Part model, mm, in its own coordinate system. Face numbers are marked on the shaded views. A direction names the side the tool comes from. Coordinates: 2 decimals unless noted, no trailing zeros. Loops run counter-clockwise (first coordinate to the right, second up) from the corner with the lowest first, then second, coordinate; pieces in that order, holes last. Notation, with made-up numbers: M 22,-28 L 52,-28 A20 ccw 52,1 Z; hole C 39.25,39 d5. An arc over 180 degrees is marked long. Use a Markdown table: item, result. Add a question column.
1) Pin check, flat tips, straight feed: pin 1 Ø1 at (y, z) = (-180, -95.5) entering from -X; pin 2 Ø12 at (y, z) = (-118.5, -103) entering from +X; pin 3 Ø14 at (x, y) = (-146, -101.5) entering from +Z. Stop position of each tip, or through.
2) Pull direction Z, two halves, no side cores. Call the marked faces 4, 5 and 6: released by +Z, released by -Z, zero draft, split by the parting line, or undercut.
3) Tool access for the marked faces 1, 2 and 3: list every direction of +Z, -Z, +X, -X, +Y, -Y with a clear straight run to the whole face (end or side of a thin tool).
4) Wall check: probe 1 along Z at (x, y) = (5.5, -134); probe 2 along Z at (x, y) = (-20, -145); probe 3 along Z at (x, y) = (-105, -100.5). Give the ranges that are in metal, low to high. Write a range as from..to.
5) Band-saw the part on D-D (x = -87). List the corners of the cut face in (y, z), plus the area to 3 significant figures.
6) Band-saw the part on B-B (x = -18.5). List the corners of the cut face in (y, z).
7) Band-saw the part on C-C (z = -47). List the corners of the cut face in (x, y), plus the area to 3 significant figures.
8) Band-saw the part on A-A (y = -166). List the corners of the cut face in (x, z), plus the area to 3 significant figures.
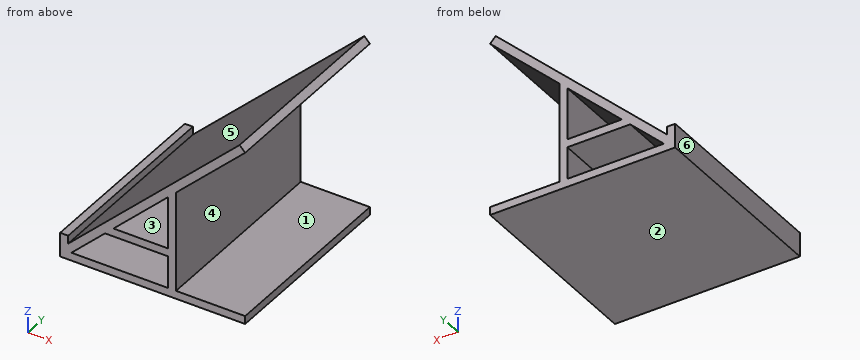
from build123d import *

# Parameters (mm, degrees)
F1_DEPTH = 304.8
F3_DEPTH = 304.8
F5_DEPTH = 304.8


with BuildPart() as f1:
    # F0 (on Front) → F1 (new body)
    with BuildSketch(Plane.XZ):
        Polygon((-139.7, -114.3), (-152.4, -114.3), (-152.4, -152.4), (-139.7, -152.4), (-139.7, -139.7), (-139.7, -127), align=None)
        Polygon((15.1285276038, 3.5224484142), (6.35, 12.7), (-139.7, -127), (-139.7, -139.7), (-134.604032102, -139.7), align=None)
        Polygon((152.4, -152.4), (152.4, -139.7), (139.7, -139.7), (-134.604032102, -139.7), (-139.7, -139.7), (-139.7, -152.4), align=None)
        Polygon((139.7, 122.6777698367), (139.7, 140.252173913), (6.35, 12.7), (15.1285276038, 3.5224484142), align=None)
        Polygon((152.4, 134.8255959236), (152.4, 152.4), (139.7, 140.252173913), (139.7, 122.6777698367), align=None)
        Polygon((152.4, -139.7), (152.4, 134.8255959236), (139.7, 122.6777698367), (139.7, -139.7), align=None)
    extrude(amount=F1_DEPTH)

    # F2 (on face) → F3 (join)
    with BuildSketch(Plane.XZ.offset(304.8)):
        Polygon((-68.2176684656, -76.2), (-81.4949411929, -88.9), (17.795967898, -88.9), (17.795967898, -76.2), align=None)
        Polygon((17.795967898, -88.9), (17.795967898, -139.7), (30.495967898, -139.7), (30.495967898, 18.2217391304), (17.795967898, 6.0739130435), (17.795967898, -76.2), align=None)
    extrude(amount=-F3_DEPTH)

    # F4 (on face) → F5 (cut)
    with BuildSketch(Plane.XZ.offset(304.8)):
        Polygon((130.9214723962, 131.8553214225), (139.7, 122.6777698367), (139.7, -139.7), (139.7, -152.4), (152.4, -152.4), (152.4, 152.4), align=None)
    extrude(amount=-F5_DEPTH, mode=Mode.SUBTRACT)


solid = f1.part
Entries:
| question | item | result |
|---|---|---|
| 1 | pin 1 | x = -107.29 |
| 1 | pin 2 | x = 30.5 |
| 1 | pin 3 | z = -114.3 |
| 2 | face 4 | undercut |
| 2 | face 5 | released by +Z |
| 2 | face 6 | zero draft |
| 3 | face 1 | +X, +Y, -Y |
| 3 | face 2 | -Z, +X, -X, +Y, -Y |
| 3 | face 3 | +Y, -Y |
| 4 | probe 1 | -152.4..-139.7, -88.9..-76.2, -5.69..11.89 |
| 4 | probe 2 | -152.4..-139.7, -88.9..-76.2, -30.08..-12.5 |
| 4 | probe 3 | -152.4..-139.7, -111.38..-93.81 |
| 5 | outline | M -304.8,-152.4 L 0,-152.4 L 0,-139.7 L -304.8,-139.7 Z; M -304.8,-94.17 L 0,-94.17 L 0,-76.59 L -304.8,-76.59 Z |
| 5 | area | 9,230 mm2 |
| 6 | outline | M -304.8,-152.4 L 0,-152.4 L 0,-139.7 L -304.8,-139.7 Z; M -304.8,-88.9 L 0,-88.9 L 0,-76.2 L -304.8,-76.2 Z; M -304.8,-28.64 L 0,-28.64 L 0,-11.07 L -304.8,-11.07 Z |
| 7 | outline | M -56.06,-304.8 L -37.69,-304.8 L -37.69,0 L -56.06,0 Z; M 17.8,-304.8 L 30.5,-304.8 L 30.5,0 L 17.8,0 Z |
| 7 | area | 9,470 mm2 |
| 8 | outline | M -152.4,-152.4 L 139.7,-152.4 L 139.7,-139.7 L 30.5,-139.7 L 30.5,18.22 L 139.7,122.68 L 130.92,131.86 L -139.7,-127 L -139.7,-114.3 L -152.4,-114.3 Z; hole M -134.6,-139.7 L 17.8,-139.7 L 17.8,-88.9 L -81.49,-88.9 Z; hole M -68.22,-76.2 L 17.8,-76.2 L 17.8,6.07 Z |
| 8 | area | 12,000 mm2 |
